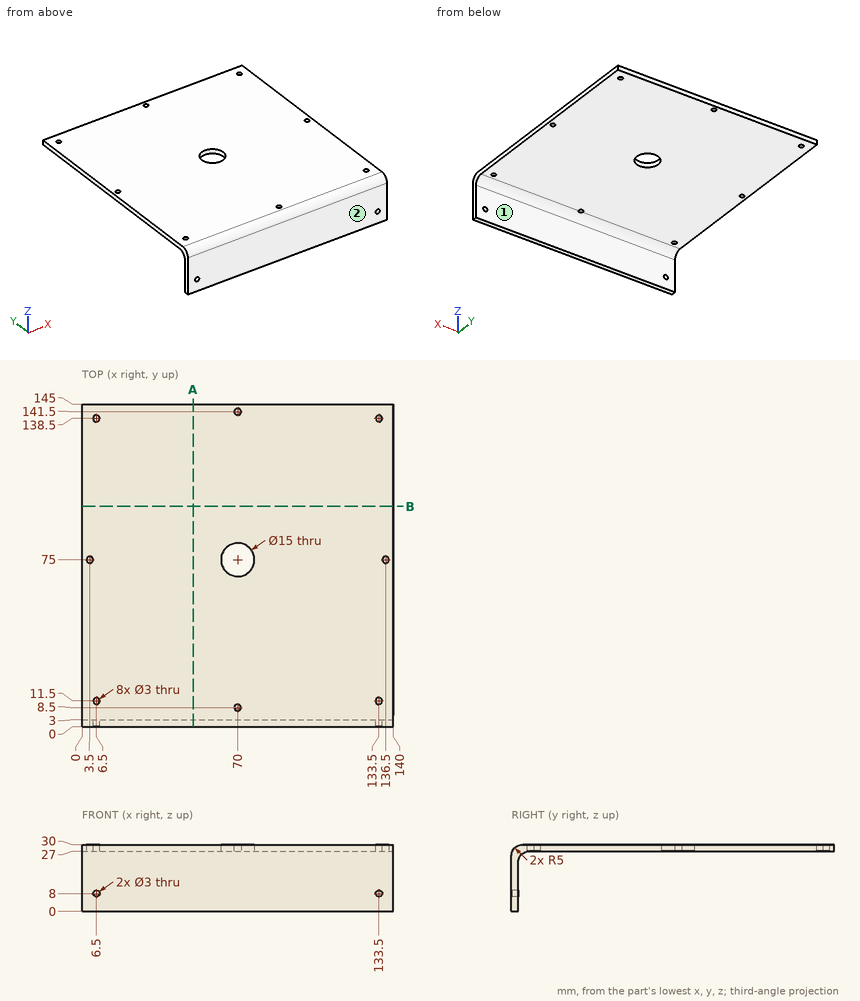
Design review of the part shown in the three views and the two pictorial views. Dimensions are in mm from the part's minimum x, y and z. A direction names the side the tool comes from. Round coordinates to 2 decimals unless told otherwise and drop trailing zeros. Loops run counter-clockwise (first coordinate to the right, second up) from the corner with the lowest first, then second, coordinate; pieces in that order, holes last.
1) Wall thickness on line 1 along X through (y, z) = (1, 8); line 2 along Y through (x, z) = (133.5, 29); line 3 along Y through (x, z) = (70, 29): over which ranges is each line inside the solid? List them lowest first.
Values follow:
line 1: x = 0 to 5, 8 to 132, 135 to 140
line 2: y = 2 to 10, 13 to 137, 140 to 145
line 3: y = 2 to 7, 10 to 67.5, 82.5 to 140, 143 to 145
2) Consider section A-A on x = 50. State the section outline as (y, z) points.
Values follow:
outline: (0, 0) - (3, 0) - (3, 22) arc R5 cw to (8, 27) - (145, 27) - (145, 30) - (5, 30) arc R5 ccw to (0, 25) - close
3) Tool access review of the marked faces 1 and 2: name each direction out of +Z, -Z, +X, -X, +Y, -Y from which nothing blocks a thin tool from reaching the whole face with its end or side.
Values follow:
face 1: -Z, +X, -X, +Y
face 2: +Z, -Z, +X, -X, -Y
4) Consider section B-B on y = 99. State the section outline as (x, z) points, then the cut area to 3 significant figures.
Values follow:
outline: (0, 27) - (140, 27) - (140, 30) - (0, 30) - close
area: 420 mm2
5) Clearance check with flat-ended pins moving along their axes: P1, Ø17, axis at x = 70, y = 75, coming from the -Z side; P2, Ø4, axis at x = 133.5, y = 138.5, coming from the +Z side; P3, Ø2.5, axis at x = 70, y = 141.5, coming from the -Z side; P4, Ø5, axis at x = 133.5, z = 8, coming from the +Y side. State where each tip first meets the part, or that it passes through.
Values follow:
P1: stops at z = 27
P2: stops at z = 30
P3: passes through
P4: stops at y = 3
